from build123d import *

# Parameters (mm, degrees)
F1_DEPTH = 3
F2_D     = 6
F3_D     = 3
F4_R     = 2


with BuildPart() as f1:
    # F0 (on Top) → F1 (new body)
    with BuildSketch(Plane.XY):
        Polygon((0, 12), (0, 0), (44, 0), (44, 12), (28, 12), (28, 18), (16, 18), (16, 12), align=None)
    extrude(amount=F1_DEPTH)

    # F2 (through all)
    with Locations(Plane(origin=(0, 0, 0), x_dir=(1, 0, 0), z_dir=(0, 0, -1))):
        with Locations((22, -12)):
            Hole(F2_D / 2)

    # F3 (through all)
    with Locations(Plane(origin=(0, 0, 0), x_dir=(1, 0, 0), z_dir=(0, 0, -1))):
        with Locations((3, -8.5), (41, -8.5)):
            Hole(F3_D / 2)

    # F4
    f4_edges = [f1.edges().sort_by_distance(p)[0] for p in [
        (28, 18, 1.5),
        (16, 18, 1.5),
        (44, 12, 1.5),
        (0, 12, 1.5),
    ]]
    fillet(f4_edges, radius=F4_R)


solid = f1.part
Could you check a few things on this model? Use its own coordinates, in mm. A direction names the side the tool comes from. Give positions to 0.01 mm unless a question says otherwise; leave off trailing zeros. Order: outer loops, then holes, each group sorted by start corner. A loop starts at its lowest first (then second) coordinate and runs counter-clockwise, first axis right, second up. Notation, with made-up numbers: (-39, 77.5) -> (0, 77.5) arc R29 cw to (0, 110.5) -> close; hole circle Ø4 at (71, 46.5). An arc over 180 degrees is marked (long way). Return JSON: item names as keys, results as strings.
1. Imagine slicing it at A-A on x = 3. List the corners of the cut face in (y, z) for me.
Answer list:
{"outline": "(0, 0) -> (7, 0) -> (7, 3) -> (0, 3) -> close; (10, 0) -> (12, 0) -> (12, 3) -> (10, 3) -> close"}
2. Thinking about a two-plate mould opening in Y: for faces 4 (the flat face through (35, 12, 1)), 5 (the flat face through (44, 5, 1)), 6 (the cylindrical face through (42.2, 9.4, 1.5)), which applies, pulls with the +Y half, pulls with the -Y half, needs draft (parallel to the pull), parting line crosses it, or undercut?
Answer list:
{"face 4": "pulls with the +Y half", "face 5": "needs draft", "face 6": "undercut"}
3. Imagine slicing it at D-D on y = 11.5. List the corners of the cut face in (x, z) for me.
Answer list:
{"outline": "(0.68, 0) -> (19.04, 0) -> (19.04, 3) -> (0.68, 3) -> close; (24.96, 0) -> (43.32, 0) -> (43.32, 3) -> (24.96, 3) -> close"}
4. For pin 1 Ø0.9 at (x, z) = (32, 1.5) entering from +Y; pin 2 Ø0.9 at (y, z) = (13.5, 2) entering from -X; pin 3 Ø1.5 at (y, z) = (14.5, 1.5) entering from +X, each with a flat end and sliding along its axis, tell me the tip position at first contact or that it passes through.
Answer list:
{"pin 1": "stops at y = 12", "pin 2": "stops at x = 16", "pin 3": "stops at x = 28"}
5. Imagine slicing it at B-B on y = 8.5. List the corners of the cut face in (x, z) for me.
Answer list:
{"outline": "(0, 0) -> (1.5, 0) -> (1.5, 3) -> (0, 3) -> close; (4.5, 0) -> (39.5, 0) -> (39.5, 3) -> (4.5, 3) -> close; (42.5, 0) -> (44, 0) -> (44, 3) -> (42.5, 3) -> close"}
6. Imagine slicing it at C-C on z = 0.75. List the corners of the cut face in (x, y) for me.
Answer list:
{"outline": "(0, 0) -> (44, 0) -> (44, 10) arc R2 ccw to (42, 12) -> (28, 12) -> (28, 16) arc R2 ccw to (26, 18) -> (18, 18) arc R2 ccw to (16, 16) -> (16, 12) -> (2, 12) arc R2 ccw to (0, 10) -> close; hole circle Ø3 at (3, 8.5); hole circle Ø6 at (22, 12); hole circle Ø3 at (41, 8.5)"}
7. I need wall thicknesses on line 1 (X direction, y = 8.5, z = 0.8); line 2 (Y direction, x = 41, z = 0.3); line 3 (X direction, y = 9.5, z = 2.45). Which ranges of each line are inside material? Lowest first, please. Write a range as from..to.
Answer list:
{"line 1": "x = 0..1.5, 4.5..39.5, 42.5..44", "line 2": "y = 0..7, 10..12", "line 3": "x = 0..1.88, 4.12..20.34, 23.66..39.88, 42.12..44"}
8. On a 3-axis mill with a long thin cutter (end or side, diameter ignored), from which of +Z, -Z, +X, -X, +Y, -Y can I reach the whole of each face in a straight line? I mean faces 1 (the flat face through (22, 18, 1)), 2 (the flat face through (16, 14, 1)), 3 (the flat face through (28, 14, 1)). Say none if no direction works.
Answer list:
{"face 1": "+Z, -Z, +X, -X, +Y", "face 2": "+Z, -Z, -X, +Y", "face 3": "+Z, -Z, +X, +Y"}
